from build123d import *

# Parameters (mm, degrees)
SKETCH2_W            = 100
SKETCH2_H            = 100
BOSS_EXTRUDE1_DEPTH  = 5
SKETCH3_W            = 100
SKETCH3_H            = 100
BOSS_EXTRUDE2_DEPTH  = 5
SKETCH8_R            = 5
BOSS_EXTRUDE7_DEPTH  = 30
SKETCH9_W            = 35.4
SKETCH9_H            = 35.4
BOSS_EXTRUDE8_DEPTH  = 20
SKETCH10_W           = 25.4
SKETCH10_H           = 25.4
CUT_EXTRUDE1_DEPTH   = 12.7
SKETCH11_W           = 10
SKETCH11_H           = 10
BOSS_EXTRUDE9_DEPTH  = 20
BOSS_EXTRUDE13_DEPTH = 10
FILLET3_R            = 4
FILLET5_R            = 4
SKETCH16_W           = 10
SKETCH16_H           = 10
BOSS_EXTRUDE14_DEPTH = 20
SKETCH13_W           = 10
SKETCH13_H           = 10
BOSS_EXTRUDE11_DEPTH = 20
BOSS_EXTRUDE17_DEPTH = 10
FILLET9_R            = 4
FILLET10_R           = 4
SKETCH21_W           = 10
SKETCH21_H           = 10
BOSS_EXTRUDE18_DEPTH = 20
SKETCH14_W           = 10
SKETCH14_H           = 10
BOSS_EXTRUDE12_DEPTH = 20
BOSS_EXTRUDE15_DEPTH = 10
FILLET7_R            = 4
SKETCH18_W           = 10
SKETCH18_H           = 10
BOSS_EXTRUDE16_DEPTH = 20
FILLET8_R            = 4
SKETCH12_W           = 10
SKETCH12_H           = 10
BOSS_EXTRUDE10_DEPTH = 20
BOSS_EXTRUDE19_DEPTH = 10
FILLET11_R           = 4
FILLET12_R           = 4
SKETCH23_W           = 10
SKETCH23_H           = 10
BOSS_EXTRUDE20_DEPTH = 20


with BuildPart() as part:
    # Sketch2 → Boss-Extrude1 (new body)
    with BuildSketch(Plane(origin=(0, 0, 0), x_dir=(1, 0, 0), z_dir=(0, 1, 0))):
        Rectangle(SKETCH2_W, SKETCH2_H)
    extrude(amount=BOSS_EXTRUDE1_DEPTH)

    # Sketch3 → Boss-Extrude2 (add)
    with BuildSketch(Plane.XZ):
        Rectangle(SKETCH3_W, SKETCH3_H)
    extrude(amount=BOSS_EXTRUDE2_DEPTH)

    # Sketch8 → Boss-Extrude7 (add)
    with BuildSketch(Plane.XZ.offset(5)):
        with Locations(Location((0, 0, 0), (0, 0, 90))):
            Circle(SKETCH8_R)
    extrude(amount=BOSS_EXTRUDE7_DEPTH)

    # Sketch9 → Boss-Extrude8 (add)
    with BuildSketch(Plane.XZ.offset(35)):
        Rectangle(SKETCH9_W, SKETCH9_H)
    extrude(amount=BOSS_EXTRUDE8_DEPTH)

    # Sketch10 → Cut-Extrude1 (cut)
    with BuildSketch(Plane.XZ.offset(55)):
        Rectangle(SKETCH10_W, SKETCH10_H)
    extrude(amount=-CUT_EXTRUDE1_DEPTH, mode=Mode.SUBTRACT)

    # Sketch11 → Boss-Extrude9 (add)
    with BuildSketch(Plane(origin=(50, 0, 0), x_dir=(0, 0, -1), z_dir=(1, 0, 0))):
        Rectangle(SKETCH11_W, SKETCH11_H)
    extrude(amount=BOSS_EXTRUDE9_DEPTH)

    # Sketch15 → Boss-Extrude13 (add)
    with BuildSketch(Plane(origin=(70, 0, 0), x_dir=(0, 0, -1), z_dir=(1, 0, 0))):
        Polygon((-5, -5), (5, -5), (5, 12.5), (1, 12.5), (1, 9.5), (3, 5), (-3, 5), (-1, 9.5), (-1, 12.5), (-5, 12.5), align=None)
    extrude(amount=BOSS_EXTRUDE13_DEPTH)

    # Fillet3
    # the kernel refuses this fillet: 4 mm, written as the material it takes off along each edge
    with BuildSketch(Plane(origin=(60.317541634, 12.5, 1), x_dir=(0, -1, 0), z_dir=(1, 0, 0))) as fillet3_piece_1:
        with BuildLine():
            CenterArc((4, -3.872983346), FILLET3_R, 104.477512186, 75.522487814)
            Line((0, -3.872983346), (-0.08, -3.872983346))
            Line((-0.08, -3.872983346), (-0.08, 0))
            Line((-0.08, 0), (0, 0.08))
            ThreePointArc((0, 0.08), (1.5, 0.08), (2.98, 0.077459667))
            Line((2.98, 0.077459667), (3, 0))
        make_face()
    extrude(amount=29.364916731, mode=Mode.SUBTRACT)

    # Fillet5
    # the kernel refuses this fillet: 4 mm, written as the material it takes off along each edge
    with BuildSketch(Plane(origin=(60.317541634, 12.5, -1), x_dir=(0, 0, -1), z_dir=(1, 0, 0))) as fillet5_piece_1:
        with BuildLine():
            CenterArc((3.872983346, -4), FILLET5_R, 90, 75.522487814)
            Line((0, -3), (-0.077459667, -2.98))
            ThreePointArc((-0.077459667, -2.98), (-0.08, -1.5), (-0.08, 0))
            Line((-0.08, 0), (0, 0.08))
            Line((0, 0.08), (3.872983346, 0.08))
            Line((3.872983346, 0.08), (3.872983346, 0))
        make_face()
    extrude(amount=29.364916731, mode=Mode.SUBTRACT)

    # Sketch16 → Boss-Extrude14 (add)
    with BuildSketch(Plane(origin=(80, 0, 0), x_dir=(0, 0, -1), z_dir=(1, 0, 0))):
        Rectangle(SKETCH16_W, SKETCH16_H)
    extrude(amount=BOSS_EXTRUDE14_DEPTH)

    # Sketch13 → Boss-Extrude11 (add)
    with BuildSketch(Plane.ZY.offset(50)):
        Rectangle(SKETCH13_W, SKETCH13_H)
    extrude(amount=BOSS_EXTRUDE11_DEPTH)

    # Sketch19 → Boss-Extrude17 (add)
    with BuildSketch(Plane.ZY.offset(70)):
        Polygon((-5, -5), (5, -5), (5, 12.5), (1, 12.5), (1, 9.5), (3, 5), (-3, 5), (-1, 9.5), (-1, 12.499789013), (-5, 12.499789013), align=None)
    extrude(amount=BOSS_EXTRUDE17_DEPTH)

    # Fillet9
    # the kernel refuses this fillet: 4 mm, written as the material it takes off along each edge
    with BuildSketch(Plane(origin=(-60.317677841, 12.499789013, -1), x_dir=(0, -1, 0), z_dir=(-1, 0, 0))) as fillet9_piece_1:
        with BuildLine():
            CenterArc((4, -3.872928863), FILLET9_R, 104.480633491, 75.519366509)
            Line((0, -3.872928863), (-0.08, -3.872928863))
            Line((-0.08, -3.872928863), (-0.08, 0))
            Line((-0.08, 0), (0, 0.08))
            ThreePointArc((0, 0.08), (1.499894506, 0.08), (2.979784793, 0.077458577))
            Line((2.979784793, 0.077458577), (2.999789013, 0))
        make_face()
    extrude(amount=29.364644317, mode=Mode.SUBTRACT)

    # Fillet10
    # the kernel refuses this fillet: 4 mm, written as the material it takes off along each edge
    with BuildSketch(Plane(origin=(-60.317541634, 12.5, 1), x_dir=(0, 0, 1), z_dir=(-1, 0, 0))) as fillet10_piece_1:
        with BuildLine():
            CenterArc((3.872983346, -4), FILLET10_R, 90, 75.522487814)
            Line((0, -3), (-0.077459667, -2.98))
            ThreePointArc((-0.077459667, -2.98), (-0.08, -1.5), (-0.08, 0))
            Line((-0.08, 0), (0, 0.08))
            Line((0, 0.08), (3.872983346, 0.08))
            Line((3.872983346, 0.08), (3.872983346, 0))
        make_face()
    extrude(amount=29.364916731, mode=Mode.SUBTRACT)

    # Sketch21 → Boss-Extrude18 (add)
    with BuildSketch(Plane.ZY.offset(80)):
        Rectangle(SKETCH21_W, SKETCH21_H)
    extrude(amount=BOSS_EXTRUDE18_DEPTH)

    # Sketch14 → Boss-Extrude12 (add)
    with BuildSketch(Plane(origin=(0, 0, -50), x_dir=(-1, 0, 0), z_dir=(0, 0, -1))):
        Rectangle(SKETCH14_W, SKETCH14_H)
    extrude(amount=BOSS_EXTRUDE12_DEPTH)

    # Sketch17 → Boss-Extrude15 (add)
    with BuildSketch(Plane(origin=(0, 0, -70), x_dir=(-1, 0, 0), z_dir=(0, 0, -1))):
        Polygon((-5, -5), (5, -5), (5, 12.5), (1, 12.5), (1, 9.5), (3, 5), (-3, 5), (-1, 9.5), (-1, 12.5), (-5, 12.5), align=None)
    extrude(amount=BOSS_EXTRUDE15_DEPTH)

    # Fillet7
    # the kernel refuses this fillet: 4 mm, written as the material it takes off along each edge
    with BuildSketch(Plane(origin=(1, 12.5, -60.317541634), x_dir=(0, -1, 0), z_dir=(0, 0, -1))) as fillet7_piece_1:
        with BuildLine():
            CenterArc((4, -3.872983346), FILLET7_R, 104.477512186, 75.522487814)
            Line((0, -3.872983346), (-0.08, -3.872983346))
            Line((-0.08, -3.872983346), (-0.08, 0))
            Line((-0.08, 0), (0, 0.08))
            ThreePointArc((0, 0.08), (1.5, 0.08), (2.98, 0.077459667))
            Line((2.98, 0.077459667), (3, 0))
        make_face()
    extrude(amount=29.364916731, mode=Mode.SUBTRACT)

    # Sketch18 → Boss-Extrude16 (add)
    with BuildSketch(Plane(origin=(0, 0, -80), x_dir=(-1, 0, 0), z_dir=(0, 0, -1))):
        Rectangle(SKETCH18_W, SKETCH18_H)
    extrude(amount=BOSS_EXTRUDE16_DEPTH)

    # Fillet8
    # the kernel refuses this fillet: 4 mm, written as the material it takes off along each edge
    with BuildSketch(Plane(origin=(-1, 12.5, -60.317541634), x_dir=(-1, 0, 0), z_dir=(0, 0, -1))) as fillet8_piece_1:
        with BuildLine():
            CenterArc((3.872983346, -4), FILLET8_R, 90, 75.522487814)
            Line((0, -3), (-0.077459667, -2.98))
            ThreePointArc((-0.077459667, -2.98), (-0.08, -1.5), (-0.08, 0))
            Line((-0.08, 0), (0, 0.08))
            Line((0, 0.08), (3.872983346, 0.08))
            Line((3.872983346, 0.08), (3.872983346, 0))
        make_face()
    extrude(amount=29.364916731, mode=Mode.SUBTRACT)

    # Sketch12 → Boss-Extrude10 (add)
    with BuildSketch(Plane.XY.offset(50)):
        Rectangle(SKETCH12_W, SKETCH12_H)
    extrude(amount=BOSS_EXTRUDE10_DEPTH)

    # Sketch22 → Boss-Extrude19 (add)
    with BuildSketch(Plane.XY.offset(70)):
        Polygon((5, -5), (5, 12.5), (1, 12.5), (1, 9.5), (3, 5), (-3, 5), (-1, 9.5), (-1, 12.5), (-5, 12.5), (-5, -5), align=None)
    extrude(amount=BOSS_EXTRUDE19_DEPTH)

    # Fillet11
    # the kernel refuses this fillet: 4 mm, written as the material it takes off along each edge
    with BuildSketch(Plane(origin=(-1, 12.5, 60.317541634), x_dir=(0, -1, 0), z_dir=(0, 0, 1))) as fillet11_piece_1:
        with BuildLine():
            CenterArc((4, -3.872983346), FILLET11_R, 104.477512186, 75.522487814)
            Line((0, -3.872983346), (-0.08, -3.872983346))
            Line((-0.08, -3.872983346), (-0.08, 0))
            Line((-0.08, 0), (0, 0.08))
            ThreePointArc((0, 0.08), (1.5, 0.08), (2.98, 0.077459667))
            Line((2.98, 0.077459667), (3, 0))
        make_face()
    extrude(amount=29.364916731, mode=Mode.SUBTRACT)

    # Fillet12
    # the kernel refuses this fillet: 4 mm, written as the material it takes off along each edge
    with BuildSketch(Plane(origin=(1, 12.5, 60.317541634), x_dir=(1, 0, 0), z_dir=(0, 0, 1))) as fillet12_piece_1:
        with BuildLine():
            CenterArc((3.872983346, -4), FILLET12_R, 90, 75.522487814)
            Line((0, -3), (-0.077459667, -2.98))
            ThreePointArc((-0.077459667, -2.98), (-0.08, -1.5), (-0.08, 0))
            Line((-0.08, 0), (0, 0.08))
            Line((0, 0.08), (3.872983346, 0.08))
            Line((3.872983346, 0.08), (3.872983346, 0))
        make_face()
    extrude(amount=29.364916731, mode=Mode.SUBTRACT)

    # Sketch23 → Boss-Extrude20 (add)
    with BuildSketch(Plane.XY.offset(80)):
        Rectangle(SKETCH23_W, SKETCH23_H)
    extrude(amount=BOSS_EXTRUDE20_DEPTH)


solid = part.part
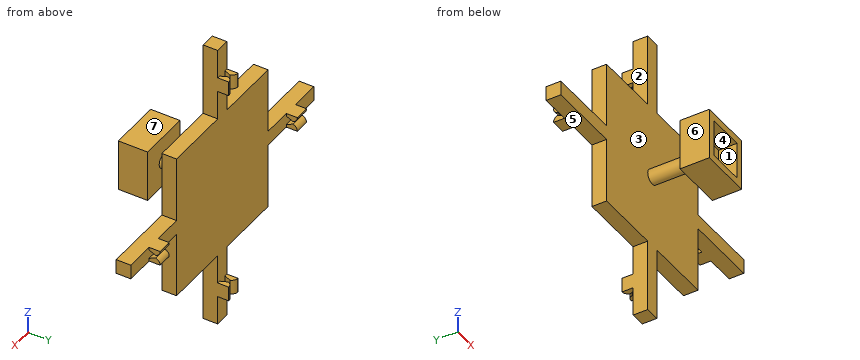
Part model, mm, in its own coordinate system. Face numbers are marked on the shaded views. A direction names the side the tool comes from. Coordinates: 2 decimals unless noted, no trailing zeros. Loops run counter-clockwise (first coordinate to the right, second up) from the corner with the lowest first, then second, coordinate; pieces in that order, holes last. Notation, with made-up numbers: (-22, 2.25) - (-13, 2.25) arc R36 ccw to (-13, 36.25) - close; hole circle Ø5 at (87, -35.5). An arc over 180 degrees is marked (long way). Write each question's results on one line, items separated by ' | '. Start each with the question number.
Q1. Drop flat-ended pins along their axis: pin 1 Ø8 at (x, y) = (34.5, 0.5) entering from -Z; pin 2 Ø12.5 at (x, z) = (-2, 2.5) entering from -Y; pin 3 Ø6 at (x, y) = (47.5, -6.5) entering from +Z. Give the stop position or say it passes through.
Q2. Probe line 1 along Z through (x, y) = (2.5, -48); line 2 along Z through (x, y) = (-28, -3); line 3 along Z through (x, y) = (74.5, 3). List the from-to ranges inside material, lowest first.
Q3. Slice it at A-A on y = -15. Give the cut face in (x, z).
Q4. Slice it at B-B on z = -61.5. Give the cut face in (x, y), and give its area (3 significant figures).
Q5. Which spindle directions (+Z, -Z, +X, -X, +Y, -Y) get a long thin tool onto all of the face, cutting with end or side? Do the marked faces 4, 5, 6 and 7. Say none if no direction does.
Q6. Two-plate mould, pull along X, no slides. Class the marked faces 1, 2 and 3: +X half, -X half, draft (parallel to the pull), parting line (faces both ways), or undercut.
Answer:
1) pin 1: stops at z = -50 | pin 2: stops at y = -42.3 | pin 3: stops at z = 50
2) line 1: z = -17.7 to -12.7, 12.7 to 17.7 | line 2: z = -50 to 50 | line 3: z = -5 to 5
3) outline: circle Ø10 at (0, 0)
4) outline: (-5, -5) - (5, -5) - (5, 5) - (-5, 5) - close | area: 100 mm2
5) face 4: -Y | face 5: -Z, -X, +Y, -Y | face 6: +Z, -Z, -X, -Y | face 7: +Z, +X, -X, -Y
6) face 1: undercut | face 2: -X half | face 3: draft
